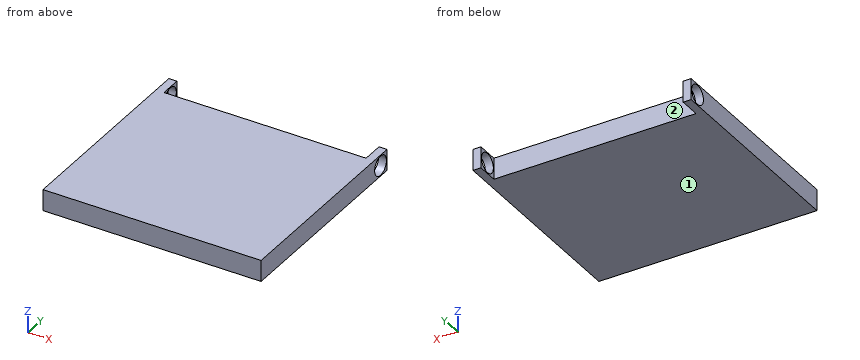
Autodesk Inventor part; units mm, degrees
ref_plane "YZ Plane" through (0, 0, 0) normal (1, 0, 0) x (0, 1, 0)
ref_plane "XZ Plane" through (0, 0, 0) normal (0, 1, 0) x (-1, 0, 0)
ref_plane "XY Plane" through (0, 0, 0) normal (0, 0, 1) x (1, 0, 0)
sketch "Sketch1" plane through (0, 0, 0) normal (0, 0, 1) x (1, 0, 0)
  line L0 (0, 0) -> (820, 0)
  line L1 (820, 0) -> (820, 700)
  line L2 (820, 700) -> (0, 700)
  line L3 (0, 700) -> (0, 0)
  dimension "d0" = 820
  dimension "d1" = 700
extrude "Extrusion1" add sketch "Sketch1" along normal blind 80
sketch "Sketch2" plane through (820, 0, 0) normal (1, 0, 0) x (0, 0, -1)
  line L0 (0, 0) -> (0, 700)
  line L1 (0, 700) -> (-80, 700)
  line L2 (-80, 0) -> (-80, 700)
  line L3 (0, 0) -> (-80, 0)
  line L4 (0, 0) -> (0, 700)
  line L5 (0, 700) -> (-80, 700)
  line L6 (-80, 700) -> (-80, 780)
  line L7 (-80, 780) -> (0, 780)
  line L8 (0, 780) -> (0, 700)
  dimension "d4" = 80
  dimension "d5" = 80
extrude "Extrusion2" add sketch "Sketch2" against normal blind 30 contours L1 L6 L7 L8
sketch "Sketch3" plane through (0, 0, 0) normal (-1, 0, 0) x (0, 0, 1)
  line L0 (0, 700) -> (0, 0)
  line L1 (0, 0) -> (80, 0)
  line L2 (80, 700) -> (80, 0)
  line L3 (0, 700) -> (80, 700)
  line L4 (0, 780) -> (0, 700)
  line L5 (80, 700) -> (0, 700)
  line L6 (80, 700) -> (80, 780)
  line L7 (80, 780) -> (0, 780)
  line L8 (80, 0) -> (80, 780)
  line L9 (0, 700) -> (80, 700)
  line L10 (80, 700) -> (80, 780)
  line L11 (80, 780) -> (0, 780)
  line L12 (0, 780) -> (0, 700)
  point P0 (72, 700)
extrude "Extrusion3" add sketch "Sketch3" against normal blind 30 contours L4 L7 L6 L3
sketch "Sketch4" plane through (0, 0, 0) normal (-1, 0, 0) x (0, 0, 1)
  line L0 (0, 780) -> (80, 780)
  line L1 (80, 780) -> (80, 700)
  line L2 (0, 700) -> (80, 700)
  line L3 (0, 700) -> (0, 780)
  circle A0 centre (40, 740) radius 36.5
  point P0 (0, 0)
  dimension "d10" = 73
extrude "Extrusion4" cut sketch "Sketch4" against normal blind 940.75 contours A0
properties part number "mesa"
Work out the finished part from the listing and answer in its coordinate system (mm). Face numbers are marked on the shaded views. Round coordinates to 2 decimals unless told otherwise and drop trailing zeros. Loops run counter-clockwise (first coordinate to the right, second up) from the corner with the lowest first, then second, coordinate; pieces in that order, holes last. Notation, with made-up numbers: (72.25, 73) -> (126.25, 73) arc R33 ccw to (126.25, 107) -> close; hole circle Ø7 at (48, 44.25). An arc over 180 degrees is marked (long way). Use one line per item in the form item = value.
(1) Find section A-A on y = 740. Give the vertices of the cut face in (x, z), then the cut area to 3 significant figures.
Answer list:
outline = (0, 0) -> (30, 0) -> (30, 3.5) -> (0, 3.5) -> close; (0, 76.5) -> (30, 76.5) -> (30, 80) -> (0, 80) -> close; (790, 0) -> (820, 0) -> (820, 3.5) -> (790, 3.5) -> close; (790, 76.5) -> (820, 76.5) -> (820, 80) -> (790, 80) -> close
area = 420 mm2
(2) For a pull along X with two mould halves and no side action, classify the marked faces 1 and 2 as released by +X, released by -X, zero draft, split by the parting line, or undercut.
Answer list:
face_1 = zero draft
face_2 = undercut
(3) Find section B-B on z = 40. Give the vertices of the cut face in (x, y), then the cut area to 3 significant figures.
Answer list:
outline = (0, 0) -> (820, 0) -> (820, 703.5) -> (790, 703.5) -> (790, 700) -> (30, 700) -> (30, 703.5) -> (0, 703.5) -> close; (0, 776.5) -> (30, 776.5) -> (30, 780) -> (0, 780) -> close; (790, 776.5) -> (820, 776.5) -> (820, 780) -> (790, 780) -> close
area = 574,000 mm2
(4) Flat-ended cylindrical pins translate along their axes: P1, Ø6, axis at y = 217, z = 53, coming from the -X side; P2, Ø1.5, axis at x = 205.5, z = 54.5, coming from the +Y side. Find the tip coordinate at first contact, or state that the pin passes through.
Answer list:
P1 = 0
P2 = 700
(5) Straight lines are drawn through the part: line 1 (Y direction, x = 806, z = 40); line 2 (Y direction, x = 724, z = 14). For each, find the intervals that lie inside material, in ascending order.
Answer list:
line_1 = 0 to 703.5, 776.5 to 780
line_2 = 0 to 700
(6) Find section C-C on x = 259. Give the vertices of the cut face in (y, z), then the cut area to 3 significant figures.
Answer list:
outline = (0, 0) -> (700, 0) -> (700, 80) -> (0, 80) -> close
area = 56,000 mm2
